CAD build for the part. Positions are in the model's coordinates, mm. A direction names the side the tool comes from. Round coordinates to 2 decimals unless told otherwise and drop trailing zeros. Loops run counter-clockwise (first coordinate to the right, second up) from the corner with the lowest first, then second, coordinate; pieces in that order, holes last. Notation, with made-up numbers: M 8,3.25 L 35,3.25 A36 ccw 35,39.25 Z; hole C 61,52.5 d8. An arc over 180 degrees is marked long. Use one line per item in the form item = value.
Autodesk Fusion 360 part; units mm, degrees
sketch "Skizze2" plane through (0, 0, 0) normal (0, 0, 1) x (1, 0, 0)
  line L0 (0, 0) -> (28.074, 0)
  line L1 (28.074, 0) -> (28.074, 76)
  line L2 (28.074, 76) -> (0, 76)
  line L3 (0, 76) -> (0, 0)
  line L4 (0, 76) -> (6, 76)
  line L5 (6, 76) -> (6, 66)
  line L6 (6, 66) -> (0, 66)
  line L7 (0, 66) -> (0, 76)
  line L8 (28.074, 76) -> (22.074, 76)
  line L9 (22.074, 76) -> (22.074, 66)
  line L10 (22.074, 66) -> (28.074, 66)
  line L11 (28.074, 66) -> (28.074, 76)
  line L12 (0, 0) -> (6, 0)
  line L13 (6, 0) -> (6, 10)
  line L14 (6, 10) -> (0, 10)
  line L15 (0, 10) -> (0, 0)
  line L16 (28.074, 0) -> (22.074, 0)
  line L17 (22.074, 0) -> (22.074, 10)
  line L18 (22.074, 10) -> (28.074, 10)
  line L19 (28.074, 10) -> (28.074, 0)
  line L20 (14.037, 76) -> (14.037, 0) construction
  line L21 (0, 20) -> (28.074, 20) construction
  line L22 (0, 56) -> (28.074, 56) construction
  circle A0 centre (14.037, 61) radius 2.25
  circle A1 centre (14.037, 51) radius 2.25
  circle A2 centre (9.037, 20) radius 2.25
  circle A3 centre (19.037, 20) radius 2.25
  line L23 (11.787, 61) -> (11.787, 51)
  line L24 (16.287, 61) -> (16.287, 51)
  line L25 (9.037, 22.25) -> (19.037, 22.25)
  line L26 (9.037, 17.75) -> (19.037, 17.75)
  line L27 (0, 76) -> (6, 76)
  line L28 (6, 76) -> (6, 71)
  line L29 (6, 71) -> (0, 71)
  line L30 (0, 71) -> (0, 76)
  line L31 (22.074, 76) -> (28.074, 76)
  line L32 (28.074, 76) -> (28.074, 71)
  line L33 (28.074, 71) -> (22.074, 71)
  line L34 (22.074, 71) -> (22.074, 76)
  line L35 (0, 10) -> (6, 10)
  line L36 (6, 10) -> (6, 5)
  line L37 (6, 5) -> (0, 5)
  line L38 (0, 5) -> (0, 10)
  line L39 (22.074, 10) -> (28.074, 10)
  line L40 (28.074, 10) -> (28.074, 5)
  line L41 (28.074, 5) -> (22.074, 5)
  line L42 (22.074, 5) -> (22.074, 10)
  point P0 (14.037, 61)
  point P1 (14.037, 51)
  point P2 (9.037, 20)
  point P3 (19.037, 20)
  point P4 (14.037, 56)
  point P5 (14.037, 20)
  dimension "d1" = 28.074
  dimension "d2" = 76
  dimension "d3" = 6
  dimension "d4" = 10
  dimension "d5" = 6
  dimension "d6" = 10
  dimension "d7" = 6
  dimension "d8" = 10
  dimension "d9" = 6
  dimension "d10" = 10
  dimension "d11" = 20
  dimension "d12" = 20
  dimension "d13" = 5
  dimension "d14" = 5
  dimension "d15" = 5
  dimension "d16" = 5
  dimension "d17" = 4.5
  dimension "d18" = 4.5
  dimension "d19" = 4.5
  dimension "d20" = 4.5
  dimension "d23" = 5
extrude "Extrusion1" add sketch "Skizze2" along normal blind 4 contours L0 L1 L2 L3 L5 L6 L9 L10 L13 L14 L17 L18 L28 L34 L35 L36 L39 L42
extrude "Extrusion2" add sketch "Skizze2" along normal blind 9 contours L0 L3 L12 L13 L15 L37 | L3 L13 L14 L15 L35 L36 L37 L38 | L0 L1 L16 L17 L19 L41 | L1 L17 L18 L19 L39 L40 L41 L42 | L3 L5 L6 L7 L29 | L2 L3 L4 L5 L7 L27 L28 L29 L30 | L1 L9 L10 L11 L33 | L1 L2 L8 L9 L11 L31 L32 L33 L34
extrude "Extrusion3" cut sketch "Skizze2" along normal blind 6.7 contours L3 L13 L14 L15 L35 L36 L37 L38 | L1 L17 L18 L19 L39 L40 L41 L42 | L2 L3 L4 L5 L7 L27 L28 L29 L30 | L1 L2 L8 L9 L11 L31 L32 L33 L34
extrude "Extrusion4" add sketch "Skizze2" along normal blind 4 contours L3 L13 L14 L15 L35 L36 L37 L38 | L1 L17 L18 L19 L39 L40 L41 L42 | L2 L3 L4 L5 L7 L27 L28 L29 L30 | L1 L2 L8 L9 L11 L31 L32 L33 L34
chamfer "Fase1" distance 3 angle 45 8 edges at (14.037, 63.25, 4) (16.287, 56, 4) (14.037, 48.75, 4) (11.787, 56, 4) (14.037, 22.25, 4) (21.287, 20, 4) (14.037, 17.75, 4) (6.787, 20, 4)
1. Pull direction X, two halves, no side cores. Call faces 6 (the face through (25, 76, 8)), 7 (the face through (22.074, 4, 7)): +X half, -X half, draft (parallel to the pull), parting line (faces both ways), or undercut.
Completed:
face_6 = draft
face_7 = undercut
2. Cut at A-A on y = 57. Write the cut outline in (x, z).
Completed:
outline = M 0,0 L 11.79,0 L 11.79,1 L 8.79,4 L 0,4 Z; M 16.29,0 L 28.07,0 L 28.07,4 L 19.29,4 L 16.29,1 Z
3. Cut at C-C on y = 8. Write the cut outline in (x, z).
Completed:
outline = M 0,0 L 28.07,0 L 28.07,4 L 0,4 Z; M 0,6.7 L 6,6.7 L 6,9 L 0,9 Z; M 22.07,6.7 L 28.07,6.7 L 28.07,9 L 22.07,9 Z
4. Probe line 1 along Y through (x, z) = (22.5, 4.5); line 2 along Y through (x, z) = (2.75, 8.25); line 3 along Z through (x, y) = (4, 34). List the from-to ranges inside material, lowest first. Write a range as from..to.
Completed:
line_1 = 0..5, 66..71
line_2 = 0..10, 66..76
line_3 = 0..4
5. Drop flat-ended pins along their axis: P1, Ø1, axis at x = 16.5, y = 62.5, coming from the +Z side; P2, Ø12, axis at x = 23, y = 33, coming from the +Z side; P3, Ø0.8, axis at x = 24, z = 5.5, coming from the +Y side. Give the stop position or say it passes through.
Completed:
P1 = 2.13
P2 = 4
P3 = 71
6. Cut at B-B on z = 5.25. Write the cut outline in (x, y), and give its area (3 significant figures).
Completed:
outline = M 0,0 L 6,0 L 6,5 L 0,5 Z; M 0,66 L 6,66 L 6,71 L 0,71 Z; M 22.07,0 L 28.07,0 L 28.07,5 L 22.07,5 Z; M 22.07,66 L 28.07,66 L 28.07,71 L 22.07,71 Z
area = 120 mm2
7. Tool access for faces 1 (the face through (22.074, 70, 7)), 2 (the face through (13.97, 47.9, 1.85)), 3 (the face through (21.286, 20.049, 0.493)), 4 (the face through (3, 74, 6.7)), 5 (the face through (3, 5, 5)): list every direction of +Z, -Z, +X, -X, +Y, -Y with a clear straight run to the whole face (end or side of a thin tool).
Completed:
face_1 = +Z, +Y, -Y
face_2 = +Z
face_3 = +Z, -Z
face_4 = +X, -X, +Y
face_5 = +X, -X
8. Cut at D-D on y = 20. Write the cut outline in (x, z), and give its area (3 significant figures).
Completed:
outline = M 0,0 L 6.79,0 L 6.79,1 L 3.79,4 L 0,4 Z; M 21.29,0 L 28.07,0 L 28.07,4 L 24.29,4 L 21.29,1 Z
area = 45.3 mm2
